Work out the finished part from the listing and answer in its coordinate system (mm). Face numbers are marked on the shaded views. A direction names the side the tool comes from. Give positions to 0.01 mm unless a question says otherwise; leave off trailing zeros. Loops run counter-clockwise (first coordinate to the right, second up) from the corner with the lowest first, then second, coordinate; pieces in that order, holes last. Notation, with made-up numbers: (-1.5, 40.5) - (50.5, 40.5) arc R18 ccw to (50.5, 68.5) - close; hole circle Ø11 at (86.5, -40). An arc over 180 degrees is marked (long way). One line per question, with ' | ' between items. Start each with the question number.
1. Find the intervals of material crossed by line 1 (X direction, y = -3.5, z = 3); line 2 (Z direction, x = -22.5, y = -13.55); line 3 (X direction, y = -13, z = 26), in increasing order.
2. Section A-A (y = -8.25) is taken. Determine the outline of the cut face in (x, z) (3 decimals).
3. Each of these flat-tipped pins is pushed along its axis until it touches: pin 1 (4 mm diameter, centred on x = -44, y = -4.5, fed in from -Z); pin 2 (0.6 mm diameter, centred on x = -0.5, y = -1, fed in from -Z); pin 3 (6 mm diameter, centred on x = -16, y = -10.5, fed in from +Z); pin 4 (5 mm diameter, centred on x = -25.9, z = 0, fed in from +Y). Where does it stop, or does it pass through?
4. Which of the six approach directions +Z, -Z, +X, -X, +Y, -Y give full straight-line access (tool end or side, diameter ignored) to the marked faces 1, 2 and 3?
5. Section B-B (x = 1.5) is taken. Give the number of separate pieces and of enclosed holes in the cut face, plus the area to 3 significant figures.
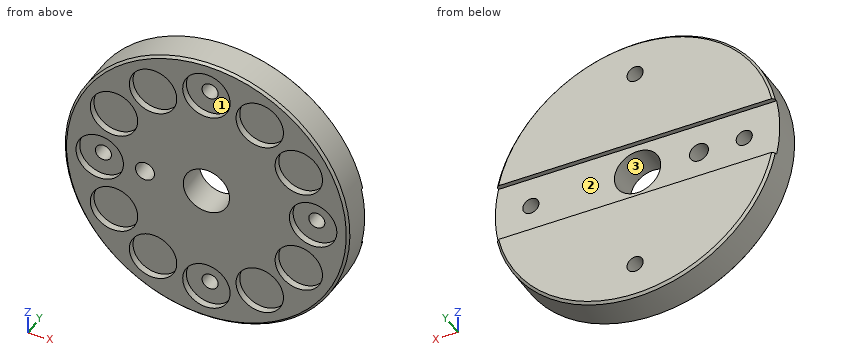
from build123d import *

# Parameters (mm, degrees)
SKETCH1_R                      = 60
SKETCH1_R_2                    = 9.765
BOSS_EXTRUDE1_DEPTH            = 15
CHAMFER1_SIZE                  = 1
M8_TAPPED_HOLE1_D              = 6.8
SKETCH5_R                      = 10
CUT_EXTRUDE1_DEPTH             = 3
CIRPATTERN1_COUNT              = 12
SKETCH7_W                      = 120
SKETCH7_H                      = 25.4
CUT_EXTRUDE2_DEPTH             = 2
CUT_EXTRUDE3_REACH             = 88.168
SKETCH8_R                      = 4
CUT_EXTRUDE3_DIRECTION_2_DEPTH = 87.168439698


with BuildPart() as part:
    # Sketch1 → Boss-Extrude1 (new body)
    with BuildSketch(Plane(origin=(0, 0, 0), x_dir=(1, 0, 0), z_dir=(0, 1, 0))):
        with Locations(Location((0, 0, 0), (0, 0, 270))):
            Circle(SKETCH1_R)
        with Locations(Location((0, 0, 0), (0, 0, 270))):
            Circle(SKETCH1_R_2, mode=Mode.SUBTRACT)
    extrude(amount=-BOSS_EXTRUDE1_DEPTH)

    # Chamfer1
    chamfer1_edges = [part.edges().sort_by_distance(p)[0] for p in [
        (0, 0, -60),
        (0, -15, -60),
    ]]
    chamfer(chamfer1_edges, length=CHAMFER1_SIZE)

    # M8 Tapped Hole1 (through all)
    with Locations(Plane(origin=(0, 0, 0), x_dir=(1, 0, 0), z_dir=(0, 1, 0))):
        with Locations((-45, 0), (0, -45), (0, 45), (45, 0)):
            Hole(M8_TAPPED_HOLE1_D / 2)

    # Sketch5 → Cut-Extrude1 (cut)
    with BuildSketch(Plane.XZ.offset(15)):
        with Locations(Location((0, 45, 0), (0, 0, 270))):
            Circle(SKETCH5_R)
    cut_extrude1 = extrude(amount=-CUT_EXTRUDE1_DEPTH, mode=Mode.SUBTRACT)

    # CirPattern1: Cut-Extrude1 ×12 about axis
    cirpattern1_axis = Axis((0, 0, 0), (0, 1, 0))
    for i in range(1, CIRPATTERN1_COUNT):
        add(cut_extrude1.rotate(cirpattern1_axis, i * 360 / CIRPATTERN1_COUNT), mode=Mode.SUBTRACT)

    # Sketch7 → Cut-Extrude2 (cut)
    with BuildSketch(Plane(origin=(0, 0, 0), x_dir=(1, 0, 0), z_dir=(0, 1, 0))):
        Rectangle(SKETCH7_W, SKETCH7_H)
    extrude(amount=-CUT_EXTRUDE2_DEPTH, mode=Mode.SUBTRACT)

    # Sketch8 → Cut-Extrude3 (cut, up to next)
    with BuildSketch(Plane(origin=(0, 0, 0), x_dir=(1, 0, 0), z_dir=(0, 1, 0)), mode=Mode.PRIVATE) as cut_extrude3_sk1:
        with Locations(Location((-25.9, 0, 0), (0, 0, 270))):
            Circle(SKETCH8_R)
    cut_extrude3_tool1 = extrude(cut_extrude3_sk1.sketch, amount=-CUT_EXTRUDE3_REACH, mode=Mode.PRIVATE) & part.part
    add(cut_extrude3_tool1.solids().sort_by_distance((-25.9, 0, 0))[0], mode=Mode.SUBTRACT)

    # Sketch8 → Cut-Extrude3 direction 2 (cut)
    with BuildSketch(Plane(origin=(0, 0, 0), x_dir=(1, 0, 0), z_dir=(0, 1, 0))):
        with Locations(Location((-25.9, 0, 0), (0, 0, 270))):
            Circle(SKETCH8_R)
    extrude(amount=CUT_EXTRUDE3_DIRECTION_2_DEPTH, mode=Mode.SUBTRACT)


solid = part.part
Conclusion:
1) line 1: -59.92 to -46.6, -43.4 to -28.55, -23.25 to -9.29, 9.29 to 43.4, 46.6 to 59.92 | line 2: -55.62 to -48.97, -28.97 to -2.11, 2.11 to 28.97, 48.97 to 55.62 | line 3: -54.07 to -48.34, -29.6 to 29.6, 48.34 to 54.07
2) outline: circle Ø120 at (0, 0); hole circle Ø6.8 at (-45, 0); hole circle Ø8 at (-25.9, 0); hole circle Ø19.53 at (0, 0); hole circle Ø6.8 at (0, -45); hole circle Ø6.8 at (0, 45); hole circle Ø6.8 at (45, 0)
3) pin 1: z = -42.85 | pin 2: z = -60 | pin 3: z = 58.57 | pin 4: through
4) face 1: -Y | face 2: +X, -X, +Y | face 3: +Y, -Y
5) separate pieces: 4 | enclosed holes: 0 | area: 1,230 mm²
